Source: CAD feature listing. Evaluate the final solid. Frame: model axes, mm. Face numbers are marked on the shaded views. A direction names the side the tool comes from. Coordinates: 2 decimals unless noted, no trailing zeros. Order: outer loops, then holes, each group sorted by start corner. A loop starts at its lowest first (then second) coordinate and runs counter-clockwise, first axis right, second up.
```python
from build123d import *

# Parameters (mm, degrees)
BOSS_EXTRUDE1_DEPTH     = 40
CUT_EXTRUDE1_DEPTH      = 49.130032204
CUT_EXTRUDE1_DEPTH_BACK = 4.1
SKETCH2_R               = 13.5
SKETCH7_R               = 11.05
CUT_EXTRUDE3_DEPTH      = 1
M5_CLEARANCE_HOLE2_D    = 5.5
FILLET1_R               = 3
SKETCH8_W               = 5
SKETCH8_H               = 40
BOSS_EXTRUDE2_DEPTH     = 3


with BuildPart() as part:
    # Sketch1 → Boss-Extrude1 (new body)
    with BuildSketch(Plane(origin=(0, 0, 0), x_dir=(1, 0, 0), z_dir=(0, 1, 0))):
        Polygon((-22.5, 14.5), (22.5, 14.5), (22.5, 11.5), (14.5, 11.5), (14.5, -14.5), (-14.5, -14.5), (-14.5, 11.5), (-22.5, 11.5), align=None)
    extrude(amount=-BOSS_EXTRUDE1_DEPTH)

    # Sketch2 → Cut-Extrude1 (cut, two sides: drawn at the far end of the back side and taken through both)
    with BuildSketch(Plane(origin=(0, 0, 0), x_dir=(1, 0, 0), z_dir=(0, 1, 0)).offset(-CUT_EXTRUDE1_DEPTH_BACK)):
        with Locations(Location((0, 0, 0), (0, 0, 270))):
            Circle(SKETCH2_R)
    extrude(amount=CUT_EXTRUDE1_DEPTH + CUT_EXTRUDE1_DEPTH_BACK, mode=Mode.SUBTRACT)

    # Sketch7 → Cut-Extrude3 (cut)
    with BuildSketch(Plane(origin=(0, -4.1, 0), x_dir=(1, 0, 0), z_dir=(0, 1, 0))):
        with Locations(Location((0, 0, 0), (0, 0, 270))):
            Circle(SKETCH7_R)
    extrude(amount=-CUT_EXTRUDE3_DEPTH, mode=Mode.SUBTRACT)

    # M5 Clearance Hole2 (through all)
    with Locations(Plane.XY.offset(-11.5)):
        with Locations((18.5, -33), (-18.5, -10), (18.5, -10), (-18.5, -33)):
            Hole(M5_CLEARANCE_HOLE2_D / 2)

    # Fillet1
    fillet1_edges = [part.edges().sort_by_distance(p)[0] for p in [
        (-14.5, -20, 14.5),
        (14.5, -20, 14.5),
    ]]
    fillet(fillet1_edges, radius=FILLET1_R)

    # Sketch8 → Boss-Extrude2 (add)
    with BuildSketch(Plane.XY.offset(-11.5)):
        with Locations((-25, -20)):
            Rectangle(SKETCH8_W, SKETCH8_H)
    extrude(amount=-BOSS_EXTRUDE2_DEPTH)


solid = part.part
```
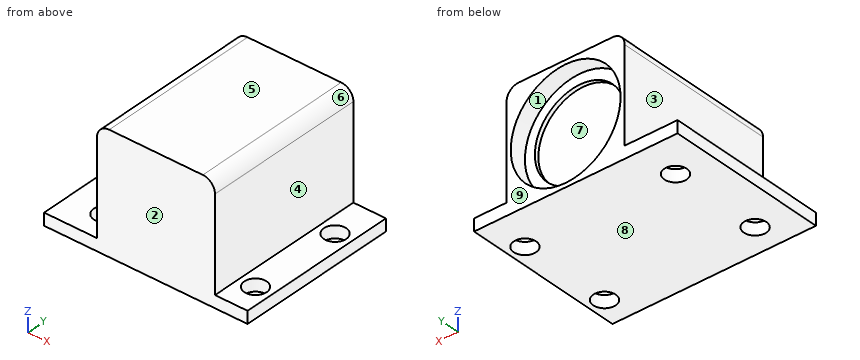
1. Ray query, line 1 (Y direction, x = 18.5, z = -12.05); line 2 (Z direction, x = 0, y = -4); line 3 (Z direction, x = -24.5, y = -22). Return the intervals inside material, ascending.
Findings:
line 1: y = -40 to -35.75, -30.25 to -12.75, -7.25 to 0
line 2: z = -14.5 to -13.5, 13.5 to 14.5
line 3: z = -14.5 to -11.5
2. Draft query along Z for the marked faces 6, 7, 8 and 9. Return one class per face: released by +Z, released by -Z, zero draft, split by the parting line, or undercut.
Findings:
face 6: released by +Z
face 7: undercut
face 8: released by -Z
face 9: zero draft
3. Section query B-B on y = -10. Return loops of the section in (x, z).
Findings:
outline: (-27.5, -14.5) - (-21.25, -14.5) - (-21.25, -11.5) - (-27.5, -11.5) - close; (-15.75, -14.5) - (15.75, -14.5) - (15.75, -11.5) - (14.5, -11.5) - (14.5, 11.5) arc R3 ccw to (11.5, 14.5) - (-11.5, 14.5) arc R3 ccw to (-14.5, 11.5) - (-14.5, -11.5) - (-15.75, -11.5) - close; (21.25, -14.5) - (22.5, -14.5) - (22.5, -11.5) - (21.25, -11.5) - close
4. Pin query (flat end, axial travel): P1, Ø6.5, axis at x = 19, y = -27.5, coming from the +Z side; P2, Ø9, axis at x = 18.5, y = -33, coming from the +Z side; P3, Ø11.5, axis at y = -20, z = -2, coming from the -X side; P4, Ø4, axis at x = -19, y = -10.5, coming from the +Z side. Return the tip coordinate at first contact, or that it passes through.
Findings:
P1: stops at z = -11.5
P2: stops at z = 13.16
P3: stops at x = -14.5
P4: passes through
5. Section query A-A on y = -3.5. Return loops of the section in (x, z).
Findings:
outline: (-27.5, -14.5) - (22.5, -14.5) - (22.5, -11.5) - (14.5, -11.5) - (14.5, 11.5) arc R3 ccw to (11.5, 14.5) - (-11.5, 14.5) arc R3 ccw to (-14.5, 11.5) - (-14.5, -11.5) - (-27.5, -11.5) - close; hole circle Ø27 at (0, 0)
6. Section query D-D on x = 0. Return loops of the section in (y, z).
Findings:
outline: (-40, -14.5) - (0, -14.5) - (0, -13.5) - (-4.1, -13.5) - (-4.1, -11.05) - (-5.1, -11.05) - (-5.1, 11.05) - (-4.1, 11.05) - (-4.1, 13.5) - (0, 13.5) - (0, 14.5) - (-40, 14.5) - close
7. Access query for the marked faces 1, 2, 3, 4 and 5. Directions: +Z, -Z, +X, -X, +Y, -Y. A direction counts if a zero-diameter tool reaches every point of the face in a straight line with its end or side. Return the directions, or none.
Findings:
face 1: +Y
face 2: +Z, -Z, +X, -X, -Y
face 3: +Z, -X, +Y, -Y
face 4: +Z, +X, +Y, -Y
face 5: +Z, +X, -X, +Y, -Y
8. Section query C-C on x = 18.5. Return loops of the section in (y, z).
Findings:
outline: (-40, -14.5) - (-35.75, -14.5) - (-35.75, -11.5) - (-40, -11.5) - close; (-30.25, -14.5) - (-12.75, -14.5) - (-12.75, -11.5) - (-30.25, -11.5) - close; (-7.25, -14.5) - (0, -14.5) - (0, -11.5) - (-7.25, -11.5) - close
